```python
from build123d import *

# Parameters (mm, degrees)
SKETCH1_W           = 101.6
SKETCH1_H           = 50.8
BOSS_EXTRUDE1_DEPTH = 6
SKETCH2_W           = 50.8
SKETCH2_H           = 40.64
CUT_EXTRUDE1_DEPTH  = 5.5
SKETCH3_R           = 1.63195
CUT_EXTRUDE2_DEPTH  = 58.112170332
SKETCH4_R           = 1.63195
CUT_EXTRUDE3_DEPTH  = 58.112170332


with BuildPart() as part:
    # Sketch1 → Boss-Extrude1 (new body)
    with BuildSketch(Plane(origin=(0, 0, 0), x_dir=(1, 0, 0), z_dir=(0, 1, 0))):
        Rectangle(SKETCH1_W, SKETCH1_H)
    extrude(amount=BOSS_EXTRUDE1_DEPTH)

    # Sketch2 → Cut-Extrude1 (cut)
    with BuildSketch(Plane(origin=(0, 6, 0), x_dir=(1, 0, 0), z_dir=(0, 1, 0))):
        Rectangle(SKETCH2_W, SKETCH2_H)
    extrude(amount=-CUT_EXTRUDE1_DEPTH, mode=Mode.SUBTRACT)

    # Sketch3 → Cut-Extrude2 (cut, through all)
    with BuildSketch(Plane(origin=(0, 6, 0), x_dir=(1, 0, 0), z_dir=(0, 1, 0))):
        with Locations(Location((-33.1, 0, 0), (0, 0, 270))):
            Circle(SKETCH3_R)
    extrude(amount=-CUT_EXTRUDE2_DEPTH, mode=Mode.SUBTRACT)

    # Sketch4 → Cut-Extrude3 (cut, through all)
    with BuildSketch(Plane(origin=(0, 6, 0), x_dir=(1, 0, 0), z_dir=(0, 1, 0))):
        with Locations(Location((33.1, 0, 0), (0, 0, 270))):
            Circle(SKETCH4_R)
    extrude(amount=-CUT_EXTRUDE3_DEPTH, mode=Mode.SUBTRACT)


solid = part.part
```
Here's how the part is built. I have some questions about the finished solid (model axes, mm). A direction names the side the tool comes from. Coordinates: 2 decimals unless noted, no trailing zeros. Order: outer loops, then holes, each group sorted by start corner. A loop starts at its lowest first (then second) coordinate and runs counter-clockwise, first axis right, second up. Notation, with made-up numbers: (62.5, 37) - (116.5, 37) arc R35 cw to (116.5, 69) - close; hole circle Ø11 at (83, 72.25). An arc over 180 degrees is marked (long way). One line per question, with ' | ' between items. Start each with the question number.
1. If we section it at D-D (y = 1.45): Write out the boundary of the cut face in (x, z), and give its area (3 significant figures).
2. I'm going to push a flat-ended pin straight in: pin 1 Ø2 at (x, z) = (33.1, 0) entering from +Y. Where does the tip first touch, or does it pass through?
3. If we section it at C-C (z = 8.5): Write out the boundary of the cut face in (x, y), and give its area (3 significant figures).
4. Which directions (+Z, -Z, +X, -X, +Y, -Y) give clear straight access to the entire face, cutting with the end or side of a thin tool? Please do faces 1 (the flat face through (-1, 6, 22)), 2 (the flat face through (25.4, 3, 0)).
5. Please list where these lines run through material, in increasing order: line 1 along X through (y, z) = (3.9, 0); line 2 along Z through (x, y) = (21, 2.35); line 3 along X through (y, z) = (2.3, 12.5). Write a range as [from, to].
6. If we mould it in two halves opening along Z, with no side actions, what happens to faces 3 (the flat face through (-1, 3, -25.4)), 4 (the flat face through (0, 0.5, 0)), 5 (the flat face through (50.8, 3, 0))? For each: released by +Z, released by -Z, zero draft, split by the parting line, or undercut.
7. If we section it at B-B (x = 33.1): Write out the boundary of the cut face in (y, z).
8. If we section it at A-A (z = 0): Write out the boundary of the cut face in (x, y), and give its area (3 significant figures).
Model answer:
1) outline: (-50.8, -25.4) - (50.8, -25.4) - (50.8, 25.4) - (-50.8, 25.4) - close; hole circle Ø3.26 at (-33.1, 0); hole (-25.4, -20.32) - (25.4, -20.32) - (25.4, 20.32) - (-25.4, 20.32) - close; hole circle Ø3.26 at (33.1, 0) | area: 3,080 mm²
2) pin 1: passes through
3) outline: (-50.8, 0) - (50.8, 0) - (50.8, 6) - (25.4, 6) - (25.4, 0.5) - (-25.4, 0.5) - (-25.4, 6) - (-50.8, 6) - close | area: 330 mm²
4) face 1: +Z, -Z, +X, -X, +Y | face 2: +Y
5) line 1: x = [-50.8, -34.73], [-31.47, -25.4], [25.4, 31.47], [34.73, 50.8] | line 2: z = [-25.4, -20.32], [20.32, 25.4] | line 3: x = [-50.8, -25.4], [25.4, 50.8]
6) face 3: released by -Z | face 4: undercut | face 5: zero draft
7) outline: (0, -25.4) - (6, -25.4) - (6, -1.63) - (0, -1.63) - close; (0, 1.63) - (6, 1.63) - (6, 25.4) - (0, 25.4) - close
8) outline: (-50.8, 0) - (-34.73, 0) - (-34.73, 6) - (-50.8, 6) - close; (-31.47, 0) - (31.47, 0) - (31.47, 6) - (25.4, 6) - (25.4, 0.5) - (-25.4, 0.5) - (-25.4, 6) - (-31.47, 6) - close; (34.73, 0) - (50.8, 0) - (50.8, 6) - (34.73, 6) - close | area: 291 mm²
